Study the drawing (mm; zero at the part's minimum x, y, z) and answer. A direction names the side the tool comes from. Coordinates: 2 decimals unless noted, no trailing zeros. Order: outer loops, then holes, each group sorted by start corner. A loop starts at its lowest first (then second) coordinate and runs counter-clockwise, first axis right, second up. Notation, with made-up numbers: M 3,-29 L 54,-29 A4 ccw 54,-25 Z; hole C 82,-12.75 d5. An arc over 180 degrees is marked long. Use a Markdown table: item, result. Add a question column.
1) For the marked faces 1, 2, 3 and 4, determine the directions among +Z, -Z, +X, -X, +Y, -Y from which every point of the face is accessible in a straight line to the end or side of a thin tool.
2) Each of these flat-tipped pins is pushed along its axis until it touches: pin 1 Ø3 at (x, z) = (81.5, 7) entering from -Y; pin 2 Ø0.6 at (x, z) = (38.5, 1) entering from -Y; pin 3 Ø3 at (x, y) = (57.5, 42) entering from +Z (3 decimals); pin 4 Ø1 at (y, z) = (97.5, 0.5) entering from -X. Where does it stop, or does it pass through?
3) Find section D-D on y = 33. Write down the section's boundary in (x, z) (3 decimals).
4) Find section B-B on z = 6.5. Write down the section's boundary in (x, y) (3 decimals), plus the area to 3 significant figures.
5) Find the intervals of material crossed by probe 1 along X at (y, z) = (56, 9.75) (3 decimals); probe 2 along X at (y, z) = (42, 0.5) (3 decimals); probe 3 along X at (y, z) = (88, 7.5), in increasing order. Write a range as [from, to].
6) Find section A-A on y = 101.5. Write down the section's boundary in (x, z) (3 decimals).
7) Find section C-C on x = 32. Write down the section's boundary in (y, z) (3 decimals), plus the area to 3 significant figures.
8) The mould has two halves that part along X. Classify the marked faces 5, 6 and 7: released by +X, released by -X, zero draft, split by the parting line, or undercut.
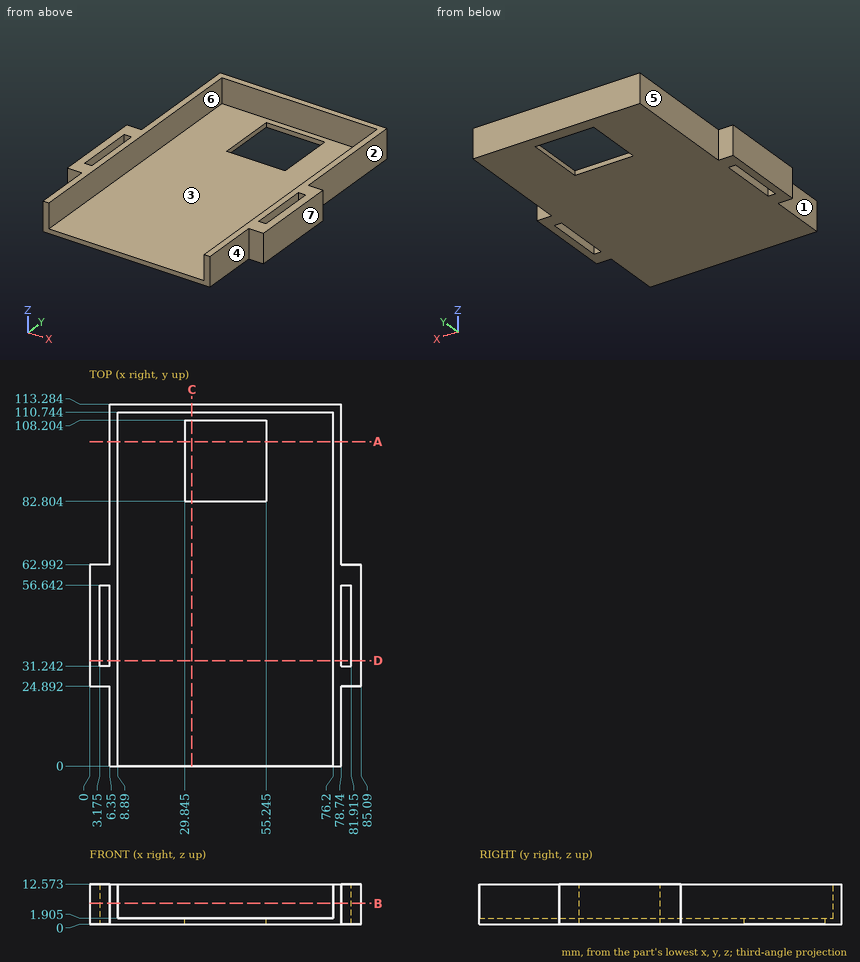
Check result:
| question | item | result |
|---|---|---|
| 1 | face 1 | +Z, -Z, -X, -Y |
| 1 | face 2 | +Z, -Z, +X, +Y |
| 1 | face 3 | +Z, -Y |
| 1 | face 4 | +Z, -Z, +X, -Y |
| 2 | pin 1 | stops at y = 24.89 |
| 2 | pin 2 | stops at y = 0 |
| 2 | pin 3 | stops at z = 1.905 |
| 2 | pin 4 | stops at x = 6.35 |
| 3 | outline | M 0,0 L 3.175,0 L 3.175,12.573 L 0,12.573 Z; M 6.35,0 L 78.74,0 L 78.74,12.573 L 76.2,12.573 L 76.2,1.905 L 8.89,1.905 L 8.89,12.573 L 6.35,12.573 Z; M 81.915,0 L 85.09,0 L 85.09,12.573 L 81.915,12.573 Z |
| 4 | outline | M 0,24.892 L 6.35,24.892 L 6.35,0 L 8.89,0 L 8.89,110.744 L 76.2,110.744 L 76.2,0 L 78.74,0 L 78.74,24.892 L 85.09,24.892 L 85.09,62.992 L 78.74,62.992 L 78.74,113.284 L 6.35,113.284 L 6.35,62.992 L 0,62.992 Z; hole M 3.175,31.242 L 6.35,31.242 L 6.35,56.642 L 3.175,56.642 Z; hole M 78.74,31.242 L 81.915,31.242 L 81.915,56.642 L 78.74,56.642 Z |
| 4 | area | 1,070 mm2 |
| 5 | probe 1 | x = [0, 3.175], [6.35, 8.89], [76.2, 78.74], [81.915, 85.09] |
| 5 | probe 2 | x = [0, 3.175], [6.35, 78.74], [81.915, 85.09] |
| 5 | probe 3 | x = [6.35, 8.89], [76.2, 78.74] |
| 6 | outline | M 6.35,0 L 29.845,0 L 29.845,1.905 L 8.89,1.905 L 8.89,12.573 L 6.35,12.573 Z; M 55.245,0 L 78.74,0 L 78.74,12.573 L 76.2,12.573 L 76.2,1.905 L 55.245,1.905 Z |
| 7 | outline | M 0,0 L 82.804,0 L 82.804,1.905 L 0,1.905 Z; M 108.204,0 L 113.284,0 L 113.284,12.573 L 110.744,12.573 L 110.744,1.905 L 108.204,1.905 Z |
| 7 | area | 195 mm2 |
| 8 | face 5 | released by -X |
| 8 | face 6 | undercut |
| 8 | face 7 | released by +X |
